Build history of the part. All positions in model axes, mm. A direction names the side the tool comes from. Coordinates: 2 decimals unless noted, no trailing zeros. Loops run counter-clockwise (first coordinate to the right, second up) from the corner with the lowest first, then second, coordinate; pieces in that order, holes last.
Item 1: Cut at C-C (y = -21). List the corners of the cut face in (x, z).
Item 2: Drill centre lines: line 1 along Y through (x, z) = (19.05, 2.5); line 2 along Y through (x, z) = (18.5, 2.25); line 3 along X through (y, z) = (74, 5.25). Where is each one in solid material? Low to high.
Item 3: Cut at D-D (y = 140.5). List the corners of the cut face in (x, z), and give its area (3 significant figures).
Item 4: Mould opens along X. For faces 1 (the face through (38.1, 83, 3)), 2 (the face through (19, 85, 6.223)), 3 (the face through (18.6, 163.8, 3.1)) say: released by +X, released by -X, zero draft, split by the parting line, or undercut.
Item 5: Cut at B-B (x = -8). List the corners of the cut face in (y, z).
Item 6: Cut at A-A (x = 19.05). List the corners of the cut face in (y, z), and give its area (3 significant figures).
Item 7: Flat gauge pins, fed straight in: pin 1 (3 mm diameter, centred on x = 48.5, z = 4.5, fed in from -Y); pin 2 (1.9 mm diameter, centred on y = 74, z = 3.5, fed in from +X). Where does each tip first touch, or does it go through?
Item 8: 3-axis set-ups, long thin cutter, end or side, ignore diameter. For faces 4 (the face through (19, 85, 0)), 5 (the face through (0, 84, 3)): which of +Z, -Z, +X, -X, +Y, -Y reach the whole face in a straight line?
from build123d import *

# Parameters (mm, degrees)
BOSS_EXTRUDE1_DEPTH = 6.223


with BuildPart() as part:
    # Sketch1 → Boss-Extrude1 (new body)
    with BuildSketch(Plane.XY):
        with BuildLine():
            ThreePointArc((0, 133.882432116), (19.05, 128.778), (38.1, 133.882432116))
            Line((38.1, 133.882432116), (38.1, 166.878))
            Line((38.1, 166.878), (22.1615, 166.878))
            ThreePointArc((22.1615, 166.878), (19.05, 163.7665), (15.9385, 166.878))
            Line((15.9385, 166.878), (0, 166.878))
            Line((0, 166.878), (0, 133.882432116))
        make_face()
        with BuildLine():
            Line((38.1, 166.878), (38.1, 133.882432116))
            ThreePointArc((38.1, 133.882432116), (52.045567884, 147.828), (57.15, 166.878))
            ThreePointArc((57.15, 166.878), (0, 199.873567884), (0, 133.882432116))
            Line((0, 133.882432116), (0, 166.878))
            Line((0, 166.878), (15.9385, 166.878))
            ThreePointArc((15.9385, 166.878), (19.05, 169.9895), (22.1615, 166.878))
            Line((22.1615, 166.878), (38.1, 166.878))
        make_face()
        with BuildLine():
            ThreePointArc((0, 32.995567884), (19.05, 38.1), (38.1, 32.995567884))
            Line((38.1, 32.995567884), (38.1, 133.882432116))
            ThreePointArc((38.1, 133.882432116), (19.05, 128.778), (0, 133.882432116))
            Line((0, 133.882432116), (0, 32.995567884))
        make_face()
        with BuildLine():
            ThreePointArc((15.9385, 0), (19.05, 3.1115), (22.1615, 0))
            Line((22.1615, 0), (38.1, 0))
            Line((38.1, 0), (38.1, 32.995567884))
            ThreePointArc((38.1, 32.995567884), (19.05, 38.1), (0, 32.995567884))
            Line((0, 32.995567884), (0, 0))
            Line((0, 0), (15.9385, 0))
        make_face()
        with BuildLine():
            Line((38.1, 0), (22.1615, 0))
            ThreePointArc((22.1615, 0), (19.05, -3.1115), (15.9385, 0))
            Line((15.9385, 0), (0, 0))
            Line((0, 0), (0, 32.995567884))
            ThreePointArc((0, 32.995567884), (0, -32.995567884), (57.15, 0))
            ThreePointArc((57.15, 0), (52.045567884, 19.05), (38.1, 32.995567884))
            Line((38.1, 32.995567884), (38.1, 0))
        make_face()
    extrude(amount=BOSS_EXTRUDE1_DEPTH)


solid = part.part
Filled sheet:
1. outline: (-12.74, 0) - (50.84, 0) - (50.84, 6.22) - (-12.74, 6.22) - close
2. line 1: y = -38.1 to -3.11, 3.11 to 163.77, 169.99 to 204.98
2. line 2: y = -38.1 to -3.06, 3.06 to 163.82, 169.94 to 204.97
2. line 3: x = 0 to 38.1
3. outline: (-8.44, 0) - (46.54, 0) - (46.54, 6.22) - (-8.44, 6.22) - close
3. area: 342 mm2
4. face 1: released by +X
4. face 2: zero draft
4. face 3: undercut
5. outline: (-26.83, 0) - (26.83, 0) - (26.83, 6.22) - (-26.83, 6.22) - close; (140.05, 0) - (193.71, 0) - (193.71, 6.22) - (140.05, 6.22) - close
6. outline: (-38.1, 0) - (-3.11, 0) - (-3.11, 6.22) - (-38.1, 6.22) - close; (3.11, 0) - (163.77, 0) - (163.77, 6.22) - (3.11, 6.22) - close; (169.99, 0) - (204.98, 0) - (204.98, 6.22) - (169.99, 6.22) - close
6. area: 1,440 mm2
7. pin 1: stops at y = -25.89
7. pin 2: stops at x = 38.1
8. face 4: -Z, +X, -X, +Y, -Y
8. face 5: +Z, -Z, -X
